Job drawing, mm, ordinate dimensions from the low corner. One solid piece. A direction names the side the tool comes from. Coordinates: 2 decimals unless noted, no trailing zeros. Loops run counter-clockwise (first coordinate to the right, second up) from the corner with the lowest first, then second, coordinate; pieces in that order, holes last. Notation, with made-up numbers: (53.5, 40) - (96.5, 40) arc R19 ccw to (96.5, 62) - close; hole circle Ø6 at (33, 84.25). An arc over 180 degrees is marked (long way). Use a Markdown table: item, result. Add a question column.
1. Band-saw the part on D-D, the plane x = 8.5. Give the cut face in (y, z).
2. Band-saw the part on B-B, the plane y = 7.5. Give the cut face in (x, z), plus the area to 3 significant figures.
3. Wall check: probe 1 along X at (y, z) = (13, 4.75); probe 2 along Z at (x, y) = (6, 7.5); probe 3 along Y at (x, z) = (7, 7.75). Give the ranges that are in metal, low to high. Write a range as [from, to].
4. Drop flat-ended pins along their axis: pin 1 (1 mm diameter, centred on x = 7.5, y = 2.5, fed in from +Z); pin 2 (3 mm diameter, centred on x = 16.5, y = 4.5, fed in from +Z); pin 3 (5 mm diameter, centred on x = 7.5, z = 11.5, fed in from +Y). Give the stop position or say it passes through.
5. 3-axis set-ups, long thin cutter, end or side, ignore diameter. For the marked faces 1 and 2: which of +Z, -Z, +X, -X, +Y, -Y reach the whole face in a straight line?
6. Band-saw the part on A-A, the plane z = 13.25. Give the cut face in (x, y), plus the area to 3 significant figures.
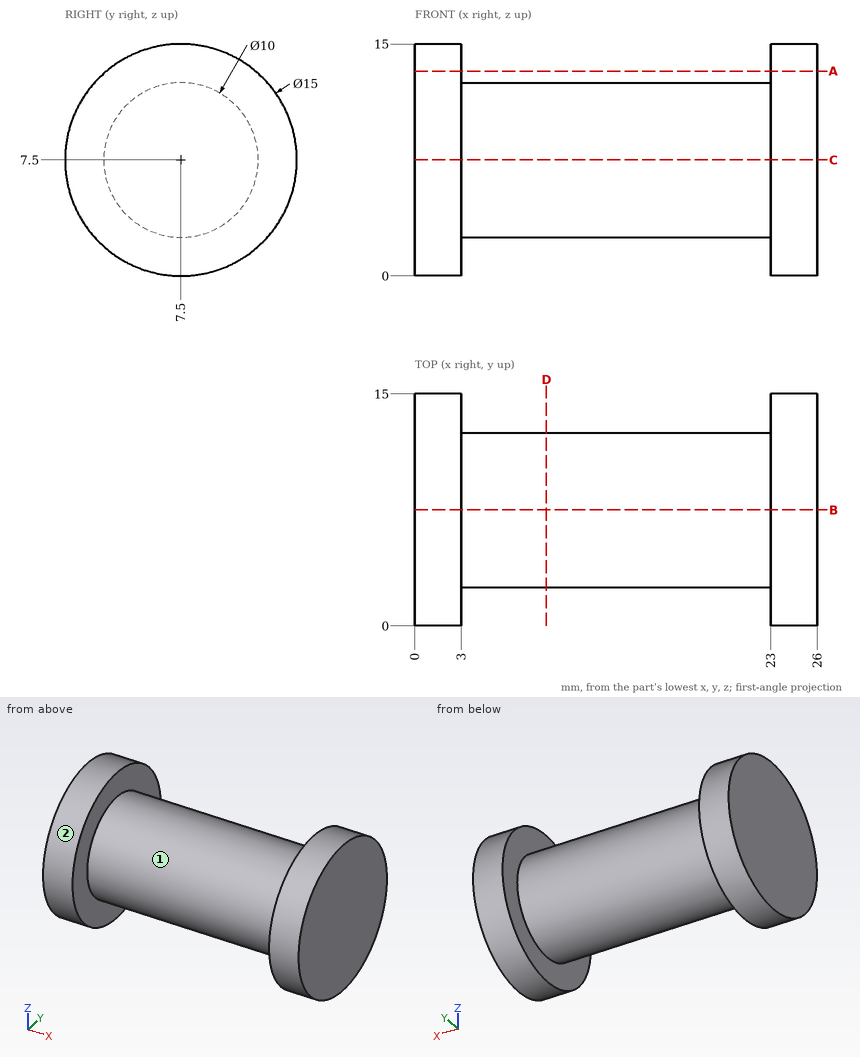
Geometry check:
| question | item | result |
|---|---|---|
| 1 | outline | circle Ø10 at (7.5, 7.5) |
| 2 | outline | (0, 0) - (3, 0) - (3, 2.5) - (23, 2.5) - (23, 0) - (26, 0) - (26, 15) - (23, 15) - (23, 12.5) - (3, 12.5) - (3, 15) - (0, 15) - close |
| 2 | area | 290 mm^2 |
| 3 | probe 1 | x = [0, 3], [23, 26] |
| 3 | probe 2 | z = [2.5, 12.5] |
| 3 | probe 3 | y = [2.51, 12.49] |
| 4 | pin 1 | stops at z = 9.68 |
| 4 | pin 2 | stops at z = 12.27 |
| 4 | pin 3 | stops at y = 12.27 |
| 5 | face 1 | none |
| 5 | face 2 | +X, -X |
| 6 | outline | (0, 2.68) - (3, 2.68) - (3, 12.32) - (0, 12.32) - close; (23, 2.68) - (26, 2.68) - (26, 12.32) - (23, 12.32) - close |
| 6 | area | 57.8 mm^2 |
